from build123d import *

# Parameters (mm, degrees)
F0_W     = 31.85
F0_H     = 23.85
F1_DEPTH = 3


with BuildPart() as f1:
    # F0 (on Top) → F1 (new body)
    with BuildSketch(Plane.XY):
        Rectangle(F0_W, F0_H)
        with BuildLine():
            Line((-11.2, -9.1), (-11.2, -10.183031))
            ThreePointArc((-11.2, -10.183031), (-12, -10.325), (-12.8, -10.183031))
            Line((-12.8, -10.183031), (-12.8, -9.1))
            ThreePointArc((-12.8, -9.1), (-12.887868, -8.887868), (-13.1, -8.8))
            Line((-13.1, -8.8), (-14.183031, -8.8))
            ThreePointArc((-14.183031, -8.8), (-14.325, -8), (-14.183031, -7.2))
            Line((-14.183031, -7.2), (-13.1, -7.2))
            ThreePointArc((-13.1, -7.2), (-12.887868, -7.112132), (-12.8, -6.9))
            Line((-12.8, -6.9), (-12.8, -5.816969))
            ThreePointArc((-12.8, -5.816969), (-12, -5.675), (-11.2, -5.816969))
            Line((-11.2, -5.816969), (-11.2, -6.9))
            ThreePointArc((-11.2, -6.9), (-11.112132, -7.112132), (-10.9, -7.2))
            Line((-10.9, -7.2), (-9.816969, -7.2))
            ThreePointArc((-9.816969, -7.2), (-9.675, -8), (-9.816969, -8.8))
            Line((-9.816969, -8.8), (-10.9, -8.8))
            ThreePointArc((-10.9, -8.8), (-11.112132, -8.887868), (-11.2, -9.1))
        make_face(mode=Mode.SUBTRACT)
        with BuildLine():
            ThreePointArc((-5.1, -7.2), (-4.887868, -7.112132), (-4.8, -6.9))
            Line((-4.8, -6.9), (-4.8, -5.816969))
            ThreePointArc((-4.8, -5.816969), (-4, -5.675), (-3.2, -5.816969))
            Line((-3.2, -5.816969), (-3.2, -6.9))
            ThreePointArc((-3.2, -6.9), (-3.112132, -7.112132), (-2.9, -7.2))
            Line((-2.9, -7.2), (-1.816969, -7.2))
            ThreePointArc((-1.816969, -7.2), (-1.675, -8), (-1.816969, -8.8))
            Line((-1.816969, -8.8), (-2.9, -8.8))
            ThreePointArc((-2.9, -8.8), (-3.112132, -8.887868), (-3.2, -9.1))
            Line((-3.2, -9.1), (-3.2, -10.183031))
            ThreePointArc((-3.2, -10.183031), (-4, -10.325), (-4.8, -10.183031))
            Line((-4.8, -10.183031), (-4.8, -9.1))
            ThreePointArc((-4.8, -9.1), (-4.887868, -8.887868), (-5.1, -8.8))
            Line((-5.1, -8.8), (-6.183031, -8.8))
            ThreePointArc((-6.183031, -8.8), (-6.325, -8), (-6.183031, -7.2))
            Line((-6.183031, -7.2), (-5.1, -7.2))
        make_face(mode=Mode.SUBTRACT)
        with BuildLine():
            Line((4.8, -9.1), (4.8, -10.183031))
            ThreePointArc((4.8, -10.183031), (4, -10.325), (3.2, -10.183031))
            Line((3.2, -10.183031), (3.2, -9.1))
            ThreePointArc((3.2, -9.1), (3.112132, -8.887868), (2.9, -8.8))
            Line((2.9, -8.8), (1.816969, -8.8))
            ThreePointArc((1.816969, -8.8), (1.675, -8), (1.816969, -7.2))
            Line((1.816969, -7.2), (2.9, -7.2))
            ThreePointArc((2.9, -7.2), (3.112132, -7.112132), (3.2, -6.9))
            Line((3.2, -6.9), (3.2, -5.816969))
            ThreePointArc((3.2, -5.816969), (4, -5.675), (4.8, -5.816969))
            Line((4.8, -5.816969), (4.8, -6.9))
            ThreePointArc((4.8, -6.9), (4.887868, -7.112132), (5.1, -7.2))
            Line((5.1, -7.2), (6.183031, -7.2))
            ThreePointArc((6.183031, -7.2), (6.325, -8), (6.183031, -8.8))
            Line((6.183031, -8.8), (5.1, -8.8))
            ThreePointArc((5.1, -8.8), (4.887868, -8.887868), (4.8, -9.1))
        make_face(mode=Mode.SUBTRACT)
        with BuildLine():
            ThreePointArc((12.8, -6.9), (12.887868, -7.112132), (13.1, -7.2))
            Line((13.1, -7.2), (14.183031, -7.2))
            ThreePointArc((14.183031, -7.2), (14.325, -8), (14.183031, -8.8))
            Line((14.183031, -8.8), (13.1, -8.8))
            ThreePointArc((13.1, -8.8), (12.887868, -8.887868), (12.8, -9.1))
            Line((12.8, -9.1), (12.8, -10.183031))
            ThreePointArc((12.8, -10.183031), (12, -10.325), (11.2, -10.183031))
            Line((11.2, -10.183031), (11.2, -9.1))
            ThreePointArc((11.2, -9.1), (11.112132, -8.887868), (10.9, -8.8))
            Line((10.9, -8.8), (9.816969, -8.8))
            ThreePointArc((9.816969, -8.8), (9.675, -8), (9.816969, -7.2))
            Line((9.816969, -7.2), (10.9, -7.2))
            ThreePointArc((10.9, -7.2), (11.112132, -7.112132), (11.2, -6.9))
            Line((11.2, -6.9), (11.2, -5.816969))
            ThreePointArc((11.2, -5.816969), (12, -5.675), (12.8, -5.816969))
            Line((12.8, -5.816969), (12.8, -6.9))
        make_face(mode=Mode.SUBTRACT)
        with BuildLine():
            ThreePointArc((-12.8, 10.183031), (-12, 10.325), (-11.2, 10.183031))
            Line((-11.2, 10.183031), (-11.2, 9.1))
            ThreePointArc((-11.2, 9.1), (-11.112132, 8.887868), (-10.9, 8.8))
            Line((-10.9, 8.8), (-9.816969, 8.8))
            ThreePointArc((-9.816969, 8.8), (-9.675, 8), (-9.816969, 7.2))
            Line((-9.816969, 7.2), (-10.9, 7.2))
            ThreePointArc((-10.9, 7.2), (-11.112132, 7.112132), (-11.2, 6.9))
            Line((-11.2, 6.9), (-11.2, 5.816969))
            ThreePointArc((-11.2, 5.816969), (-12, 5.675), (-12.8, 5.816969))
            Line((-12.8, 5.816969), (-12.8, 6.9))
            ThreePointArc((-12.8, 6.9), (-12.887868, 7.112132), (-13.1, 7.2))
            Line((-13.1, 7.2), (-14.183031, 7.2))
            ThreePointArc((-14.183031, 7.2), (-14.325, 8), (-14.183031, 8.8))
            Line((-14.183031, 8.8), (-13.1, 8.8))
            ThreePointArc((-13.1, 8.8), (-12.887868, 8.887868), (-12.8, 9.1))
            Line((-12.8, 9.1), (-12.8, 10.183031))
        make_face(mode=Mode.SUBTRACT)
        with BuildLine():
            ThreePointArc((-4.8, 10.183031), (-4, 10.325), (-3.2, 10.183031))
            Line((-3.2, 10.183031), (-3.2, 9.1))
            ThreePointArc((-3.2, 9.1), (-3.112132, 8.887868), (-2.9, 8.8))
            Line((-2.9, 8.8), (-1.816969, 8.8))
            ThreePointArc((-1.816969, 8.8), (-1.675, 8), (-1.816969, 7.2))
            Line((-1.816969, 7.2), (-2.9, 7.2))
            ThreePointArc((-2.9, 7.2), (-3.112132, 7.112132), (-3.2, 6.9))
            Line((-3.2, 6.9), (-3.2, 5.816969))
            ThreePointArc((-3.2, 5.816969), (-4, 5.675), (-4.8, 5.816969))
            Line((-4.8, 5.816969), (-4.8, 6.9))
            ThreePointArc((-4.8, 6.9), (-4.887868, 7.112132), (-5.1, 7.2))
            Line((-5.1, 7.2), (-6.183031, 7.2))
            ThreePointArc((-6.183031, 7.2), (-6.325, 8), (-6.183031, 8.8))
            Line((-6.183031, 8.8), (-5.1, 8.8))
            ThreePointArc((-5.1, 8.8), (-4.887868, 8.887868), (-4.8, 9.1))
            Line((-4.8, 9.1), (-4.8, 10.183031))
        make_face(mode=Mode.SUBTRACT)
        with BuildLine():
            ThreePointArc((3.2, 10.183031), (4, 10.325), (4.8, 10.183031))
            Line((4.8, 10.183031), (4.8, 9.1))
            ThreePointArc((4.8, 9.1), (4.887868, 8.887868), (5.1, 8.8))
            Line((5.1, 8.8), (6.183031, 8.8))
            ThreePointArc((6.183031, 8.8), (6.325, 8), (6.183031, 7.2))
            Line((6.183031, 7.2), (5.1, 7.2))
            ThreePointArc((5.1, 7.2), (4.887868, 7.112132), (4.8, 6.9))
            Line((4.8, 6.9), (4.8, 5.816969))
            ThreePointArc((4.8, 5.816969), (4, 5.675), (3.2, 5.816969))
            Line((3.2, 5.816969), (3.2, 6.9))
            ThreePointArc((3.2, 6.9), (3.112132, 7.112132), (2.9, 7.2))
            Line((2.9, 7.2), (1.816969, 7.2))
            ThreePointArc((1.816969, 7.2), (1.675, 8), (1.816969, 8.8))
            Line((1.816969, 8.8), (2.9, 8.8))
            ThreePointArc((2.9, 8.8), (3.112132, 8.887868), (3.2, 9.1))
            Line((3.2, 9.1), (3.2, 10.183031))
        make_face(mode=Mode.SUBTRACT)
        with BuildLine():
            ThreePointArc((11.2, 10.183031), (12, 10.325), (12.8, 10.183031))
            Line((12.8, 10.183031), (12.8, 9.1))
            ThreePointArc((12.8, 9.1), (12.887868, 8.887868), (13.1, 8.8))
            Line((13.1, 8.8), (14.183031, 8.8))
            ThreePointArc((14.183031, 8.8), (14.325, 8), (14.183031, 7.2))
            Line((14.183031, 7.2), (13.1, 7.2))
            ThreePointArc((13.1, 7.2), (12.887868, 7.112132), (12.8, 6.9))
            Line((12.8, 6.9), (12.8, 5.816969))
            ThreePointArc((12.8, 5.816969), (12, 5.675), (11.2, 5.816969))
            Line((11.2, 5.816969), (11.2, 6.9))
            ThreePointArc((11.2, 6.9), (11.112132, 7.112132), (10.9, 7.2))
            Line((10.9, 7.2), (9.816969, 7.2))
            ThreePointArc((9.816969, 7.2), (9.675, 8), (9.816969, 8.8))
            Line((9.816969, 8.8), (10.9, 8.8))
            ThreePointArc((10.9, 8.8), (11.112132, 8.887868), (11.2, 9.1))
            Line((11.2, 9.1), (11.2, 10.183031))
        make_face(mode=Mode.SUBTRACT)
    extrude(amount=F1_DEPTH)


solid = f1.part
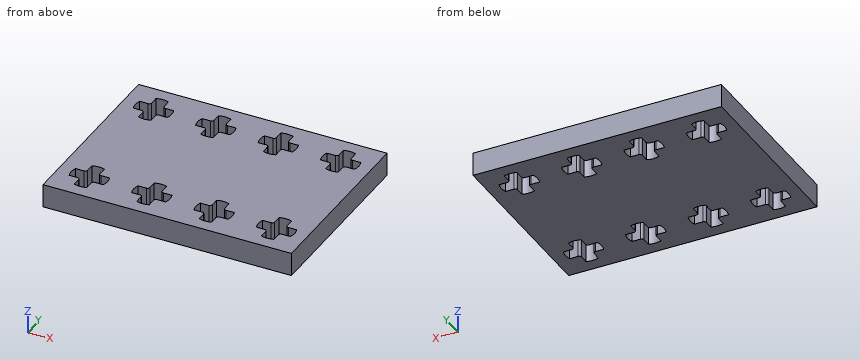
Check sheet for the modelled part. Datum: model origin and axes. Units: mm. Round coordinates to 2 decimals unless told otherwise and drop trailing zeros. Loops run counter-clockwise (first coordinate to the right, second up) from the corner with the lowest first, then second, coordinate; pieces in that order, holes last. Notation, with made-up numbers: (-1, 5.5) -> (10, 5.5) arc R26 ccw to (10, 32.5) -> close; hole circle Ø1 at (20.5, 42.5). An arc over 180 degrees is marked (long way). Put each result on its own line as item: value. Start each with the question number.
1. Scan lines: probe 1 along Y at (x, z) = (10, 2) (3 decimals); probe 2 along Y at (x, z) = (4, 0.45) (3 decimals); probe 3 along X at (y, z) = (6.75, 1.5) (3 decimals). Record each from-to range of solid material in increasing order.
2. Section check B-B (x = 12). Enter the section's corners in (y, z) (3 decimals).
3. Section check C-C (z = 0.35). Give the number of separate pieces and of enclosed holes in the cut face, plus the area to 3 significant figures.
4. Section check A-A (y = -6.25). Enter the section's corners in (x, z) (3 decimals).
Findings:
1. probe 1: y = -11.925 to -8.8, -7.2 to 7.2, 8.8 to 11.925
1. probe 2: y = -11.925 to -10.325, -5.675 to 5.675, 10.325 to 11.925
1. probe 3: x = -15.925 to -12.8, -11.2 to -4.8, -3.2 to 3.2, 4.8 to 11.2, 12.8 to 15.925
2. outline: (-11.925, 0) -> (-10.325, 0) -> (-10.325, 3) -> (-11.925, 3) -> close; (-5.675, 0) -> (5.675, 0) -> (5.675, 3) -> (-5.675, 3) -> close; (10.325, 0) -> (11.925, 0) -> (11.925, 3) -> (10.325, 3) -> close
3. separate pieces: 1
3. enclosed holes: 8
3. area: 663 mm^2
4. outline: (-15.925, 0) -> (-12.8, 0) -> (-12.8, 3) -> (-15.925, 3) -> close; (-11.2, 0) -> (-4.8, 0) -> (-4.8, 3) -> (-11.2, 3) -> close; (-3.2, 0) -> (3.2, 0) -> (3.2, 3) -> (-3.2, 3) -> close; (4.8, 0) -> (11.2, 0) -> (11.2, 3) -> (4.8, 3) -> close; (12.8, 0) -> (15.925, 0) -> (15.925, 3) -> (12.8, 3) -> close
